The listing builds one solid part. Answer for the finished solid, in the listing's coordinates (mm). A direction names the side the tool comes from. Coordinates: 2 decimals unless noted, no trailing zeros. Loops run counter-clockwise (first coordinate to the right, second up) from the corner with the lowest first, then second, coordinate; pieces in that order, holes last. Notation, with made-up numbers: (19.25, 16) -> (35.25, 16) arc R20 ccw to (35.25, 27) -> close; hole circle Ø7 at (-2, 82). An arc over 180 degrees is marked (long way). Answer in a Markdown table with one row per item.
```python
from build123d import *

# Parameters (mm, degrees)
SKETCH1_R                = 5
BOSS_EXTRUDE2_DEPTH      = 35
SKETCH3_R                = 2.5
BOSS_EXTRUDE3_DEPTH      = 5
SKETCH4_R                = 6
BOSS_EXTRUDE4_DEPTH      = 15
BOSS_EXTRUDE5_DEPTH      = 15
BOSS_EXTRUDE5_DEPTH_BACK = 15
SKETCH6_R                = 2.5
SKETCH7_R                = 6
BOSS_EXTRUDE6_DEPTH      = 10


with BuildPart() as part:
    # Sketch1 → Boss-Extrude2 (new body)
    with BuildSketch(Plane(origin=(0, 0, 0), x_dir=(0, 0, -1), z_dir=(1, 0, 0))):
        Circle(SKETCH1_R)
    extrude(amount=BOSS_EXTRUDE2_DEPTH)

    # Sketch3 → Boss-Extrude3 (add)
    with BuildSketch(Plane(origin=(35, 0, 0), x_dir=(0, 0, -1), z_dir=(1, 0, 0))):
        Circle(SKETCH3_R)
    extrude(amount=BOSS_EXTRUDE3_DEPTH)

    # Sketch4 → Boss-Extrude4 (add)
    with BuildSketch(Plane(origin=(35, 0, 0), x_dir=(0, 0, -1), z_dir=(1, 0, 0))):
        Circle(SKETCH4_R)
    extrude(amount=-BOSS_EXTRUDE4_DEPTH)

    # Sketch6 → Boss-Extrude5 (add, two sides: drawn at the far end of the back side and taken through both)
    with BuildSketch(Plane.XY.offset(-BOSS_EXTRUDE5_DEPTH_BACK)):
        with Locations((40, 0)):
            Circle(SKETCH6_R)
    extrude(amount=BOSS_EXTRUDE5_DEPTH + BOSS_EXTRUDE5_DEPTH_BACK)

    # Sketch7 → Boss-Extrude6 (add)
    with BuildSketch(Plane.ZY):
        with Locations(Location((0, 0, 0), (0, 0, 180))):
            Circle(SKETCH7_R)
    extrude(amount=BOSS_EXTRUDE6_DEPTH)


solid = part.part
```
Item 1: A cutting plane is placed at D-D, the plane y = -3.5. Determine the outline of the cut face in (x, z).
Findings below:
| item | result |
|---|---|
| outline | (-10, -4.87) -> (0, -4.87) -> (0, -3.57) -> (20, -3.57) -> (20, -4.87) -> (35, -4.87) -> (35, 4.87) -> (20, 4.87) -> (20, 3.57) -> (0, 3.57) -> (0, 4.87) -> (-10, 4.87) -> close |
Item 2: A tool of negligible diameter and unlimited length cuts with its end or side. For faces 4 (the face through (28, 0, 6)), 5 (the face through (20, 4, 4)), 6 (the face through (40, 0, -15)), from which of +Z, -Z, +X, -X, +Y, -Y can it reach the whole face along a straight path? Write none if from no direction.
Findings below:
| item | result |
|---|---|
| face 4 | -X |
| face 5 | none |
| face 6 | -Z, +X, -X, +Y, -Y |
Item 3: A cutting plane is placed at A-A, the plane z = 0. Determine the outline of the cut face in (x, y), plus the area to 3 significant figures.
Findings below:
| item | result |
|---|---|
| outline | (-10, -6) -> (0, -6) -> (0, -5) -> (20, -5) -> (20, -6) -> (35, -6) -> (35, -2.5) -> (40, -2.5) arc R2.5 ccw to (40, 2.5) -> (35, 2.5) -> (35, 6) -> (20, 6) -> (20, 5) -> (0, 5) -> (0, 6) -> (-10, 6) -> close |
| area | 535 mm2 |
Item 4: Determine the mould class of faces 1 (the face through (-10, 0, 0)), 2 (the face through (-4.93, -1.802, -5.723)), 3 (the face through (35, 0, -3)) for opening direction X: +X half, -X half, draft (parallel to the pull), parting line (faces both ways), or undercut.
Findings below:
| item | result |
|---|---|
| face 1 | -X half |
| face 2 | draft |
| face 3 | undercut |
Item 5: A cutting plane is placed at B-B, the plane y = 0. Determine the outline of the cut face in (x, z), plus the area to 4 significant figures.
Findings below:
| item | result |
|---|---|
| outline | (-10, -6) -> (0, -6) -> (0, -5) -> (20, -5) -> (20, -6) -> (35, -6) -> (35, -2.5) -> (37.5, -2.5) -> (37.5, -15) -> (42.5, -15) -> (42.5, 15) -> (37.5, 15) -> (37.5, 2.5) -> (35, 2.5) -> (35, 6) -> (20, 6) -> (20, 5) -> (0, 5) -> (0, 6) -> (-10, 6) -> close |
| area | 662.5 mm2 |
Item 6: Flat-ended cylindrical pins translate along their axes: pin 1 Ø4 at (x, y) = (31, -0.5) entering from +Z; pin 2 Ø3 at (x, y) = (-1.5, 2.5) entering from -Z. Find the tip coordinate at first contact, or state that the pin passes through.
Findings below:
| item | result |
|---|---|
| pin 1 | stops at z = 6 |
| pin 2 | stops at z = -5.92 |
Item 7: A cutting plane is placed at C-C, the plane x = 39.5. Determine the outline of the cut face in (y, z).
Findings below:
| item | result |
|---|---|
| outline | (-2.45, -15) -> (2.45, -15) -> (2.45, -0.5) arc R2.5 ccw to (2.45, 0.5) -> (2.45, 15) -> (-2.45, 15) -> (-2.45, 0.5) arc R2.5 ccw to (-2.45, -0.5) -> close |
Item 8: Find the intervals of material crossed by probe 1 along X at (y, z) = (3.25, -4); probe 2 along Z at (x, y) = (2, 0); probe 3 along X at (y, z) = (-3.5, -0.5), in increasing order.
Findings below:
| item | result |
|---|---|
| probe 1 | x = -10 to 0, 20 to 35 |
| probe 2 | z = -5 to 5 |
| probe 3 | x = -10 to 35 |
